Input: part model. Units: mm. Frame: model coordinates. Round coordinates to 2 decimals unless told otherwise and drop trailing zeros. Loops run counter-clockwise (first coordinate to the right, second up) from the corner with the lowest first, then second, coordinate; pieces in that order, holes last. Notation, with made-up numbers: (55.25, -11) -> (87.25, -11) arc R26 ccw to (87.25, 23) -> close; hole circle Ø3 at (69, 33.5). An arc over 180 degrees is marked (long way). Answer as a JSON object with one key per item and string values. Group by question number.
Item 1: Section query A-A on x = 3.5. Return loops of the section in (y, z).
Item 2: Draft query along Z for faces 1 (the cylindrical face through (12.11, -2.22, 3.03)), 2 (the flat face through (-6, 12, -17.5)), 3 (the cylindrical face through (11.916, 15.836, -20.035)), 4 (the cylindrical face through (-26.259, 1.503, -21.548)). Return one class per face: released by +Z, released by -Z, zero draft, split by the parting line, or undercut.
Item 3: Pin query (flat end, axial travel): pin 1 (7.5 mm diameter, centred on x = -20, z = -10.6, fed in from -Y); pin 2 (8 mm diameter, centred on x = -14, z = 2, fed in from +Y); pin 3 (21 mm diameter, centred on x = 12, y = 20.5, fed in from +Z). Return the tip coordinate at first contact, or that it passes through.
Item 4: Section query D-D on y = 24. Return loops of the section in (x, z).
Item 5: Section query C-C on x = -7.5. Return loops of the section in (y, z), and give its area (3 significant figures).
Item 6: Section query B-B on y = 9. Return loops of the section in (x, z), and give its area (3 significant figures).
Item 7: Material intervals for line 1 (Y direction, x = 0, z = -18); line 2 (Z direction, x = 9.5, y = -3.35) (3 decimals); line 3 (X direction, y = -1.2, z = 1.95) (3 decimals), sorted ascending. Write a range as [from, to].
from build123d import *

# Parameters (mm, degrees)
SKETCH1_W           = 64
SKETCH1_H           = 45
SKETCH1_R           = 1.6
SKETCH1_R_2         = 2.825
SKETCH1_R_3         = 4.75
BOSS_EXTRUDE1_DEPTH = 4.5
CHAMFER1_SIZE       = 1.5
BOSS_EXTRUDE2_START = -22.5
SKETCH2_R           = 10.25
SKETCH2_R_2         = 1.6
BOSS_EXTRUDE2_DEPTH = 5
FILLET1_R           = 5
FILLET2_R           = 10


with BuildPart() as part:
    # Sketch1 → Boss-Extrude1 (new body)
    with BuildSketch(Plane(origin=(0, 0, 0), x_dir=(1, 0, 0), z_dir=(0, 1, 0))):
        Rectangle(SKETCH1_W, SKETCH1_H)
        with Locations((-1.5, 8.15)):
            Circle(SKETCH1_R, mode=Mode.SUBTRACT)
        with Locations((-19, -10.75)):
            Circle(SKETCH1_R, mode=Mode.SUBTRACT)
        with Locations((9.5, -1.95)):
            Circle(SKETCH1_R_2, mode=Mode.SUBTRACT)
        with Locations((23.5, -1.95)):
            Circle(SKETCH1_R_2, mode=Mode.SUBTRACT)
        with Locations((-20, 10.6)):
            Circle(SKETCH1_R_3, mode=Mode.SUBTRACT)
        with Locations((20, 10.6)):
            Circle(SKETCH1_R_3, mode=Mode.SUBTRACT)
    extrude(amount=-BOSS_EXTRUDE1_DEPTH)

    # Chamfer1
    chamfer1_edges = [part.edges().sort_by_distance(p)[0] for p in [
        (-3.1, 0, -8.15),
        (-20.6, 0, 10.75),
    ]]
    chamfer(chamfer1_edges, length=CHAMFER1_SIZE)

    # Sketch2 → Boss-Extrude2 (add)
    with BuildSketch(Plane.XY.offset(BOSS_EXTRUDE2_START)):
        with BuildLine():
            Line((-27, 0), (-20.654878501, 26.243845624))
            ThreePointArc((-20.654878501, 26.243845624), (0, 42.5), (20.654878501, 26.243845624))
            Line((20.654878501, 26.243845624), (27, 0))
            Line((27, 0), (27, -4.5))
            Line((27, -4.5), (-27, -4.5))
            Line((-27, -4.5), (-27, 0))
        make_face()
        with Locations((0, 21.25)):
            Circle(SKETCH2_R, mode=Mode.SUBTRACT)
        with Locations((0, 35.25)):
            Circle(SKETCH2_R_2, mode=Mode.SUBTRACT)
        with Locations((-7.5, 34.240381057)):
            Circle(SKETCH2_R_2, mode=Mode.SUBTRACT)
        with Locations((12.124355653, 14.25)):
            Circle(SKETCH2_R_2, mode=Mode.SUBTRACT)
        with Locations((15, 21.25)):
            Circle(SKETCH2_R_2, mode=Mode.SUBTRACT)
        with Locations((-12.124355653, 14.25)):
            Circle(SKETCH2_R_2, mode=Mode.SUBTRACT)
        with Locations((-7.5, 8.259618943)):
            Circle(SKETCH2_R_2, mode=Mode.SUBTRACT)
    extrude(amount=BOSS_EXTRUDE2_DEPTH)

    # Fillet1
    fillet1_edges = [part.edges().sort_by_distance(p)[0] for p in [
        (32, -2.25, 22.5),
        (-32, -2.25, 22.5),
    ]]
    fillet(fillet1_edges, radius=FILLET1_R)

    # Fillet2
    fillet2_edges = [part.edges().sort_by_distance(p)[0] for p in [
        (32, -2.25, -22.5),
        (-32, -2.25, -22.5),
    ]]
    fillet(fillet2_edges, radius=FILLET2_R)


solid = part.part
Solved:
{
 "1": {"outline": "(-4.5, -22.5) -> (11.62, -22.5) -> (11.62, -17.5) -> (0, -17.5) -> (0, 22.5) -> (-4.5, 22.5) -> close; (30.88, -22.5) -> (42.21, -22.5) -> (42.21, -17.5) -> (30.88, -17.5) -> close"},
 "2": {"face 1": "undercut", "face 2": "released by +Z", "face 3": "zero draft", "face 4": "released by -Z"},
 "3": {"pin 1": "through", "pin 2": "y = 0", "pin 3": "z = -17.5"},
 "4": {"outline": "(-21.2, -22.5) -> (-9.87, -22.5) -> (-9.87, -17.5) -> (-21.2, -17.5) -> close; (9.87, -22.5) -> (21.2, -22.5) -> (21.2, -17.5) -> (9.87, -17.5) -> close"},
 "5": {"outline": "(-4.5, -22.5) -> (6.66, -22.5) -> (6.66, -17.5) -> (0, -17.5) -> (0, 22.5) -> (-4.5, 22.5) -> close; (9.86, -22.5) -> (14.26, -22.5) -> (14.26, -17.5) -> (9.86, -17.5) -> close; (28.24, -22.5) -> (32.64, -22.5) -> (32.64, -17.5) -> (28.24, -17.5) -> close; (35.84, -22.5) -> (41.13, -22.5) -> (41.13, -17.5) -> (35.84, -17.5) -> close", "area": "306 mm²"},
 "6": {"outline": "(-24.82, -22.09) arc R10 ccw to (-22, -22.5) -> (-8.92, -22.5) -> (-8.92, -17.5) -> (-24.82, -17.5) -> close; (-6.08, -22.5) -> (22, -22.5) arc R10 ccw to (24.82, -22.09) -> (24.82, -17.5) -> (-6.08, -17.5) -> close", "area": "233 mm²"},
 "7": {"line 1": "[-4.5, 11], [31.5, 33.65], [36.85, 42.5]", "line 2": "[-22.5, -0.875], [4.775, 22.5]", "line 3": "[-32, 6.675], [12.325, 20.675], [26.325, 32]"}
}
